Work out the finished part from the listing and answer in its coordinate system (mm). A direction names the side the tool comes from. Give positions to 0.01 mm unless a question says otherwise; leave off trailing zeros. Loops run counter-clockwise (first coordinate to the right, second up) from the corner with the lowest first, then second, coordinate; pieces in that order, holes last. Notation, with made-up numbers: (-3, 16) - (31, 16) arc R16 ccw to (31, 25) - close; hole circle Ø10 at (-15, -14.75). An arc over 180 degrees is marked (long way). Use CSV: the item, a comma, the result in double quotes.
from build123d import *

# Parameters (mm, degrees)
F0_W     = 10
F0_H     = 4
F0_W_2   = 23.5
F1_DEPTH = 3
F2_DEPTH = 10


with BuildPart() as f1:
    # F0 (on Top) → F1 (new body)
    with BuildSketch(Plane.XY):
        Polygon((-10.75, -35), (-10.75, 0), (10.75, 0), (10.75, -35), (34.25, -35), (34.25, 0), (55.75, 0), (55.75, -35), (65.75, -35), (65.75, 10), (-20.75, 10), (-20.75, -35), align=None)
        with Locations((-15.75, -37)):
            Rectangle(F0_W, F0_H)
        with Locations((22.5, -37)):
            Rectangle(F0_W_2, F0_H)
        with Locations((60.75, -37)):
            Rectangle(F0_W, F0_H)
    extrude(amount=F1_DEPTH)

    # F0 (on Top) → F2 (join)
    with BuildSketch(Plane.XY):
        with Locations((-15.75, -37)):
            Rectangle(F0_W, F0_H)
        with Locations((22.5, -37)):
            Rectangle(F0_W_2, F0_H)
        with Locations((60.75, -37)):
            Rectangle(F0_W, F0_H)
    extrude(amount=-F2_DEPTH)


solid = f1.part
Item 1: A cutting plane is placed at B-B on z = -7.5. Determine the outline of the cut face in (x, y), and give its area (3 significant figures).
Determined:
outline,"(-20.75, -39) - (-10.75, -39) - (-10.75, -35) - (-20.75, -35) - close; (10.75, -39) - (34.25, -39) - (34.25, -35) - (10.75, -35) - close; (55.75, -39) - (65.75, -39) - (65.75, -35) - (55.75, -35) - close"
area,"174 mm²"
Item 2: A cutting plane is placed at D-D on x = 30. Determine the outline of the cut face in (y, z).
Determined:
outline,"(-39, -10) - (-35, -10) - (-35, 0) - (10, 0) - (10, 3) - (-39, 3) - close"
Item 3: Given P1, Ø2.5, axis at x = 44, z = 2, coming from the -Y side; P2, Ø3, axis at x = 58.5, z = -7.5, coming from the +Y side; P3, Ø6, axis at x = 21.5, y = -30.5, coming from the -Z side, each flat-ended and moving along its own axis, determine where each tip first touches the part or whether it passes through.
Determined:
P1,"stops at y = 0"
P2,"stops at y = -35"
P3,"stops at z = 0"
Item 4: For faces 4 (the flat face through (-16, -39, -3)), 5 (the flat face through (45, 0, 1)), 6 (the flat face through (61, -35, -5)), determine the directions among +Z, -Z, +X, -X, +Y, -Y from which every point of the face is accessible in a straight line to the end or side of a thin tool.
Determined:
face 4,"+Z, -Z, +X, -X, -Y"
face 5,"+Z, -Z, -Y"
face 6,"-Z, +X, -X, +Y"
Item 5: A cutting plane is placed at A-A on y = -32.5. Determine the outline of the cut face in (x, z).
Determined:
outline,"(-20.75, 0) - (-10.75, 0) - (-10.75, 3) - (-20.75, 3) - close; (10.75, 0) - (34.25, 0) - (34.25, 3) - (10.75, 3) - close; (55.75, 0) - (65.75, 0) - (65.75, 3) - (55.75, 3) - close"
Item 6: Find the intervals of material crossed by line 1 (Z direction, x = 20, y = -2.5); line 2 (Y direction, x = 29.5, z = -3.75); line 3 (Y direction, x = 44, z = 1.25), in increasing order.
Determined:
line 1,"z = 0 to 3"
line 2,"y = -39 to -35"
line 3,"y = 0 to 10"
Item 7: The mould has two halves that part along X. Classify faces 1 (the flat face through (0, 0, 1)), 2 (the flat face through (-16, -37, -10)), 3 (the flat face through (-20.75, -20.1, 0.4)): pulls with the +X half, pulls with the -X half, needs draft (parallel to the pull), parting line crosses it, or undercut.
Determined:
face 1,"undercut"
face 2,"needs draft"
face 3,"pulls with the -X half"
Item 8: A cutting plane is placed at C-C on z = 1.75. Determine the outline of the cut face in (x, y).
Determined:
outline,"(-20.75, -39) - (-10.75, -39) - (-10.75, 0) - (10.75, 0) - (10.75, -39) - (34.25, -39) - (34.25, 0) - (55.75, 0) - (55.75, -39) - (65.75, -39) - (65.75, 10) - (-20.75, 10) - close"
